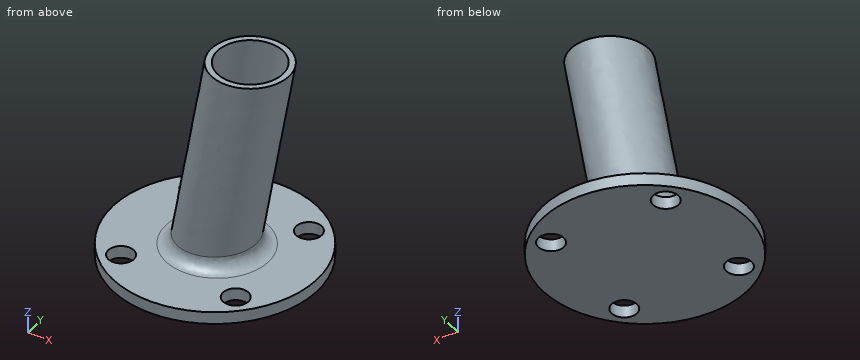
Autodesk Inventor part; units mm, degrees
ref_plane "YZ Plane" through (0, 0, 0) normal (1, 0, 0) x (0, 1, 0)
ref_plane "XZ Plane" through (0, 0, 0) normal (0, 1, 0) x (-1, 0, 0)
ref_plane "XY Plane" through (0, 0, 0) normal (0, 0, 1) x (1, 0, 0)
sketch "Sketch2" plane through (0, 0, 0) normal (0, 0, 1) x (-1, 0, 0)
  circle A0 centre (0, 0) radius 25
  line L0 (0, 0) -> (20, 0) construction
  line L1 (0, 0) -> (20, 0) construction
  line L2 (0, 0) -> (20, 0) construction
  line L3 (0, 0) -> (20, 0) construction
  circle A1 centre (14.1421, 14.1421) radius 3.125
  circle A2 centre (-14.1421, 14.1421) radius 3.125
  circle A3 centre (-14.1421, -14.1421) radius 3.125
  circle A4 centre (14.1421, -14.1421) radius 3.125
  dimension "d0" = 50
  dimension "d10" = 6.25
  dimension "d11" = 6.25
  dimension "d12" = 6.25
  dimension "d13" = 6.25
extrude "Extrusion1" add sketch "Sketch2" along normal blind 3
sketch "Sketch19" plane through (0, 0, 3) normal (0, 0, 1) x (1, 0, 0)
  circle A0 centre (0, 0) radius 9.5
  dimension "d40" = 19
sketch "Sketch22" plane through (0, 0, 0) normal (0, 1, 0) x (-1, 0, 0)
  line L0 (25, 3) -> (-25, 3)
  line L1 (0, 3) -> (-8.6824, 52.2404)
  line L2 (0, 3) -> (50, 3) construction
  point P0 (0, 0)
  dimension "d41" = 50
  dimension "d42" = 100
sweep "Sweep4" add profiles "Sketch19" path "Sketch22" path curves L1
sketch "Sketch23" plane through (0, 0, 3) normal (0, 0, 1) x (1, 0, 0)
  circle A0 centre (0, 0) radius 8
  dimension "d45" = 16
sketch "Sketch25" plane through (0, 0, 0) normal (0, 1, 0) x (-1, 0, 0)
  line L0 (25, 3) -> (-25, 3)
  line L1 (0, 3) -> (-8.6824, 52.2404)
  line L2 (0, 3) -> (50, 3) construction
  point P0 (0, 0)
  dimension "d46" = 50
  dimension "d47" = 100
sweep "Sweep5" cut profiles "Sketch23" path "Sketch25" path curves L1
fillet "Fillet2" radius 3 1 edges at (-9.5, 0, 3)
properties part number "SoporteMarcador"
Build history of the part. All positions in model axes, mm. Coordinates: 2 decimals unless noted, no trailing zeros. Order: outer loops, then holes, each group sorted by start corner. A loop starts at its lowest first (then second) coordinate and runs counter-clockwise, first axis right, second up. Notation, with made-up numbers: (83.5, -28.5) -> (105.5, -28.5) arc R34 ccw to (105.5, 9.5) -> close; hole circle Ø3 at (84.5, -33.75). An arc over 180 degrees is marked (long way). Answer in a Markdown table with one row per item. Add a question column.
Q1. Wall check: line 1 along Z through (x, y) = (-7, 22.5); line 2 along Y through (x, z) = (5, 28); line 3 along X through (y, z) = (-3.5, 25). Give the ranges that are in metal, low to high. Write a range as [from, to].
Q2. Drop flat-ended pins along their axis: pin 1 (10 mm diameter, centred on y = -18.5, z = 9.5, fed in from -X); pin 2 (5 mm diameter, centred on x = 0.5, z = 7, fed in from -Y); pin 3 (10 mm diameter, centred on x = -14.14, y = 14.14, fed in from +Z); pin 4 (4 mm diameter, centred on x = -3, z = 21, fed in from -Y). Give the stop position or say it passes through.
Q3. Band-saw the part on A-A, the plane y = 18.5. List the corners of the cut face in (x, z), then the cut area to 3 significant figures.
Answers follow:
| question | item | result |
|---|---|---|
| 1 | line 1 | [0, 3] |
| 1 | line 2 | [-9.48, -7.98], [7.98, 9.48] |
| 1 | line 3 | [-4.95, -3.31], [11.07, 12.71] |
| 2 | pin 1 | through |
| 2 | pin 2 | y = -9.9 |
| 2 | pin 3 | z = 3 |
| 2 | pin 4 | y = -8.55 |
| 3 | outline | (-16.82, 0) -> (16.82, 0) -> (16.82, 3) -> (-16.82, 3) -> close |
| 3 | area | 101 mm^2 |
